Answer from the drawing. Dimensions are ordinates in mm from the lowest x, y and z of the part. Coordinates: 2 decimals unless noted, no trailing zeros. Write each loop counter-clockwise with the first axis right and the second up, starting at its lowest first coordinate (ties: lowest second). Pieces come first, ordered by that corner, then holes.
(1) The part is cut by section C-C on z = 1.95. Give the number of separate pieces and of enclosed holes in the cut face, plus the area to 3 significant figures.
(2) The part is cut by section A-A on y = 62.5. Determine the outline of the cut face in (x, z).
(3) The part is cut by section B-B on x = 17.5. Determine the outline of the cut face in (y, z), plus the area to 3 significant figures.
(4) Straight lines are drawn through the part: line 1 (Y direction, x = 17.5, z = 2.4); line 2 (X direction, y = 32, z = 0.75) (1 decimal); line 3 (Y direction, x = 53, z = 1.25) (1 decimal). For each, find the intervals that lie inside material, in ascending order.
(5) Given P1, Ø23.5, axis at x = 69.46, y = 32.5, coming from the -Z side; P2, Ø1, axis at y = 25, z = 0.5, coming from the -X side, each flat-ended and moving along its own axis, determine where each tip first touches the part or whether it passes through.
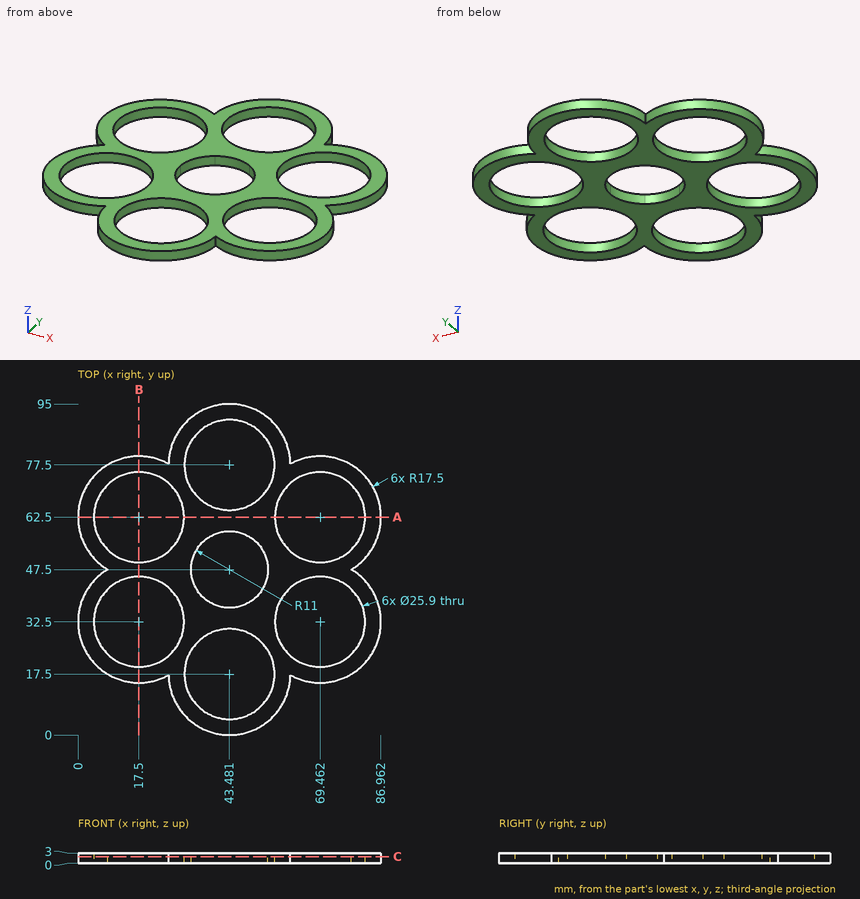
Model answer:
1. separate pieces: 1
1. enclosed holes: 7
1. area: 2,460 mm2
2. outline: (0, 0) - (4.55, 0) - (4.55, 3) - (0, 3) - close; (30.45, 0) - (56.51, 0) - (56.51, 3) - (30.45, 3) - close; (82.41, 0) - (86.96, 0) - (86.96, 3) - (82.41, 3) - close
3. outline: (15, 0) - (19.55, 0) - (19.55, 3) - (15, 3) - close; (45.45, 0) - (49.55, 0) - (49.55, 3) - (45.45, 3) - close; (75.45, 0) - (80, 0) - (80, 3) - (75.45, 3) - close
3. area: 39.6 mm2
4. line 1: y = 15 to 19.55, 45.45 to 49.55, 75.45 to 80
4. line 2: x = 0 to 4.6, 30.4 to 56.5, 82.4 to 87
4. line 3: y = 2.8 to 8.7, 26.3 to 42, 53 to 68.7, 86.3 to 92.2
5. P1: passes through
5. P2: stops at x = 1.46
